The model under review builds one solid part; all positions refer to its coordinate system, in mm. Coordinates: 2 decimals unless noted, no trailing zeros. Write each loop counter-clockwise with the first axis right and the second up, starting at its lowest first coordinate (ties: lowest second). Pieces come first, ordered by that corner, then holes. Notation, with made-up numbers: (44.5, 39.25) -> (63.5, 39.25) arc R20 cw to (63.5, 49.25) -> close; hole circle Ø9 at (12.25, 0). An arc over 180 degrees is marked (long way). Put each result on its own line as item: value. Start each with the question number.
from build123d import *

# Parameters (mm, degrees)
SKETCH_1_R          = 2.2
EXTRUDE_1_DEPTH     = 5
SKETCH_2_R          = 3.3
CUT_EXTRUDE_1_DEPTH = 10


with BuildPart() as part:
    # 草图1 → 凸台-拉伸1 (new body)
    with BuildSketch(Plane.XY):
        Polygon((-200, 150), (200, 150), (200, 110), (205, 110), (205, 70), (200, 70), (200, 30), (205, 30), (205, -30), (200, -30), (200, -70), (205, -70), (205, -110), (200, -110), (200, -150), (160, -150), (160, -155), (120, -155), (120, -150), (80, -150), (80, -155), (40, -155), (40, -150), (-40, -150), (-40, -155), (-80, -155), (-80, -150), (-120, -150), (-120, -155), (-160, -155), (-160, -150), (-200, -150), (-200, -110), (-205, -110), (-205, -70), (-200, -70), (-200, -30), (-205, -30), (-205, 30), (-200, 30), (-200, 70), (-205, 70), (-205, 110), (-200, 110), align=None)
        with Locations((-140, -140)):
            Circle(SKETCH_1_R, mode=Mode.SUBTRACT)
        with Locations((-100, -140)):
            Circle(SKETCH_1_R, mode=Mode.SUBTRACT)
        with Locations((-60, -140)):
            Circle(SKETCH_1_R, mode=Mode.SUBTRACT)
        with Locations((-20, -140)):
            Circle(SKETCH_1_R, mode=Mode.SUBTRACT)
        with Locations((20, -140)):
            Circle(SKETCH_1_R, mode=Mode.SUBTRACT)
        with Locations((60, -140)):
            Circle(SKETCH_1_R, mode=Mode.SUBTRACT)
        with Locations((100, -140)):
            Circle(SKETCH_1_R, mode=Mode.SUBTRACT)
        with Locations((140, -140)):
            Circle(SKETCH_1_R, mode=Mode.SUBTRACT)
        with Locations((-190, 110)):
            Circle(SKETCH_1_R, mode=Mode.SUBTRACT)
        with Locations((-190, 70)):
            Circle(SKETCH_1_R, mode=Mode.SUBTRACT)
        with Locations((-190, 30)):
            Circle(SKETCH_1_R, mode=Mode.SUBTRACT)
        with Locations((-190, -30)):
            Circle(SKETCH_1_R, mode=Mode.SUBTRACT)
        with Locations((-190, -70)):
            Circle(SKETCH_1_R, mode=Mode.SUBTRACT)
        with Locations((-190, -110)):
            Circle(SKETCH_1_R, mode=Mode.SUBTRACT)
        with Locations((190, -110)):
            Circle(SKETCH_1_R, mode=Mode.SUBTRACT)
        with Locations((190, -70)):
            Circle(SKETCH_1_R, mode=Mode.SUBTRACT)
        with Locations((190, -30)):
            Circle(SKETCH_1_R, mode=Mode.SUBTRACT)
        with Locations((190, 30)):
            Circle(SKETCH_1_R, mode=Mode.SUBTRACT)
        with Locations((190, 70)):
            Circle(SKETCH_1_R, mode=Mode.SUBTRACT)
        with Locations((190, 110)):
            Circle(SKETCH_1_R, mode=Mode.SUBTRACT)
    extrude(amount=EXTRUDE_1_DEPTH)

    # 草图2 → 切除-拉伸1 (cut)
    with BuildSketch(Plane.XY.offset(5)):
        with Locations((-80, 130.5)):
            Circle(SKETCH_2_R)
        with Locations((-128, 130.5)):
            Circle(SKETCH_2_R)
        with Locations((128, 130.5)):
            Circle(SKETCH_2_R)
        with Locations((80, 130.5)):
            Circle(SKETCH_2_R)
    extrude(amount=-CUT_EXTRUDE_1_DEPTH, mode=Mode.SUBTRACT)


solid = part.part
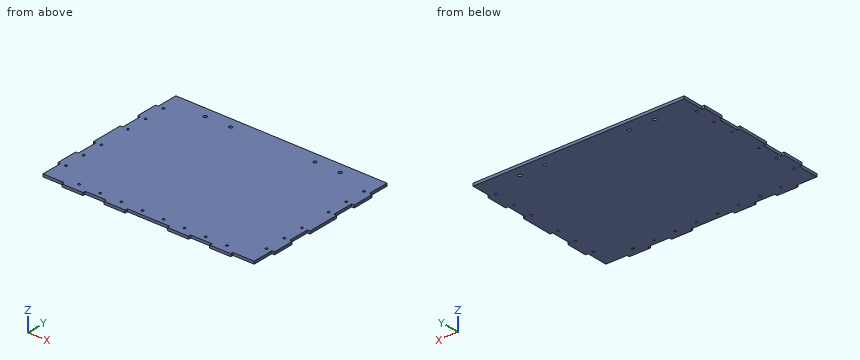
1. Consider section B-B on y = -55.5. State the section outline as (x, z) points.
2. Consider section A-A on z = 1.1. State how many separate pieces and enclosed holes the cut face has, then the cut area to 3 significant figures.
3. Insertion check: P1, Ø5.5, axis at x = 80, y = 130.5, coming from the -Z side; P2, Ø1.5, axis at y = -152, z = 2.5, coming from the -X side; P3, Ø2.5, axis at y = -152, z = 3.5, coming from the +X side; P4, Ø1.5, axis at x = 203.5, z = 3.5, coming from the +Y side. Each pin has a flat end and moves straight along its axis. Give the tip position at first contact, or say it passes through.
4. Wall thickness on line 1 (X direction, y = 130.5, z = 1.55); line 2 (Y direction, x = -100, z = 3.3); line 3 (X direction, y = 72, z = 2.2): over which ranges is each line inside the solid? List them lowest first. Write a range as from..to.
Output values:
1. outline: (-200, 0) -> (200, 0) -> (200, 5) -> (-200, 5) -> close
2. separate pieces: 1
2. enclosed holes: 24
2. area: 122,000 mm^2
3. P1: passes through
3. P2: stops at x = -160
3. P3: stops at x = 160
3. P4: stops at y = 110
4. line 1: x = -200..-131.3, -124.7..-83.3, -76.7..76.7, 83.3..124.7, 131.3..200
4. line 2: y = -150..-142.2, -137.8..150
4. line 3: x = -205..-190.92, -189.08..189.08, 190.92..205
